Part model, mm, in its own coordinate system. Face numbers are marked on the shaded views. Coordinates: 2 decimals unless noted, no trailing zeros. Loops run counter-clockwise (first coordinate to the right, second up) from the corner with the lowest first, then second, coordinate; pieces in that order, holes last. Notation, with made-up numbers: (25, -38.75) - (52, -38.75) arc R37 ccw to (52, -0.75) - close; hole circle Ø3 at (79.5, 48). An arc over 180 degrees is marked (long way). Use a Markdown table: item, result. Add a question column.
1. Drop flat-ended pins along their axis: pin 1 (0.8 mm diameter, centred on x = -0.5, y = 17.5, fed in from -Z); pin 2 (4 mm diameter, centred on x = -45, z = 17.5, fed in from -Y); pin 3 (1 mm diameter, centred on x = 17, y = 8, fed in from +Z). Give the stop position or say it passes through.
2. Wall check: probe 1 along X at (y, z) = (4.25, 1.5); probe 2 along Y at (x, z) = (-23.5, -43.5); probe 3 along X at (y, z) = (2, -8). Give the ranges that are in metal, low to high. Write a range as [from, to].
3. Band-saw the part on A-A, the plane y = 10.5. Give the cut face in (x, z).
4. Pull direction Z, two halves, no side cores. Call the marked faces 1 and 2: pulls with the +Z half, pulls with the -Z half, needs draft (parallel to the pull), parting line crosses it, or undercut.
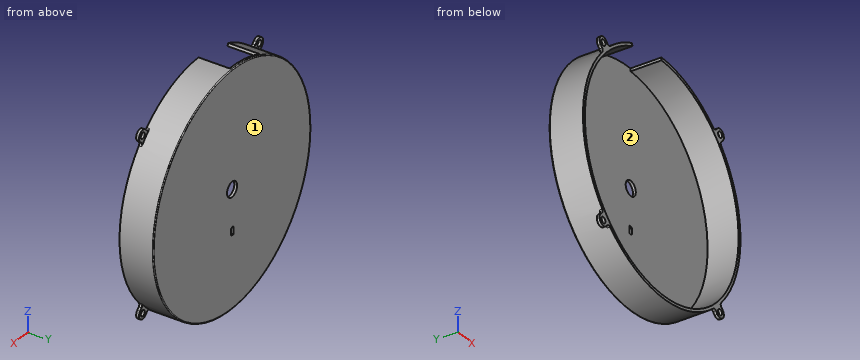
from build123d import *

# Parameters (mm, degrees)
EXTRUDE_1_DEPTH = 16.5
SKETCH_2_R      = 4
EXTRUDE_2_DEPTH = 1.5
FILLET_1_R      = 0.5
SKETCH_3_R      = 1.6
EXTRUDE_4_DEPTH = 1.5
FILLET_2_R      = 1.5


with BuildPart() as part:
    # Эскиз1 → Бобышка-Вытянуть1 (new body)
    with BuildSketch(Plane(origin=(0, 0, 0), x_dir=(1, 0, 0), z_dir=(0, 1, 0))):
        with BuildLine():
            Line((-23.77906371, -57.799706998), (-23.205036867, -56.41388361))
            ThreePointArc((-23.205036867, -56.41388361), (11.826941696, 59.842488669), (0, -61))
            Line((0, -61), (-0.15, -61))
            Line((-0.15, -61), (-0.15, -62.49982))
            ThreePointArc((-0.15, -62.49982), (12.193145126, 61.299080025), (-23.77906371, -57.799706998))
        make_face()
    extrude(amount=EXTRUDE_1_DEPTH)

    # Эскиз2 → Бобышка-Вытянуть2 (add)
    # profile 1 of 2: a face of its own
    with BuildSketch(Plane(origin=(0, 16.5, 0), x_dir=(1, 0, 0), z_dir=(0, 1, 0))):
        with BuildLine():
            Line((0, -61), (-0.15, -61))
            Line((-0.15, -61), (-0.15, -62.49982))
            ThreePointArc((-0.15, -62.49982), (12.193145126, 61.299080025), (-23.77906371, -57.799706998))
            Line((-23.77906371, -57.799706998), (-23.205036867, -56.41388361))
            ThreePointArc((-23.205036867, -56.41388361), (11.826941696, 59.842488669), (0, -61))
        make_face()
    # profile 2 of 2: a face of its own
    with BuildSketch(Plane(origin=(0, 16.5, 0), x_dir=(1, 0, 0), z_dir=(0, 1, 0))):
        with BuildLine():
            Line((-23.205036867, -56.41388361), (-23.77906371, -57.799706998))
            ThreePointArc((-23.77906371, -57.799706998), (-12.193145126, -61.299080025), (-0.15, -62.49982))
            Line((-0.15, -62.49982), (-0.15, -61))
            Line((-0.15, -61), (0, -61))
            ThreePointArc((0, -61), (11.826941696, 59.842488669), (-23.205036867, -56.41388361))
        make_face()
        with Locations(Location((0, 0, 0), (0, 0, 270))):
            Circle(SKETCH_2_R, mode=Mode.SUBTRACT)
        Polygon((-1, 23.5), (-1, 24.05), (-0.25, 24.05), (1, 23.5), (1, 20.3), (-0.25, 19.75), (-1, 19.75), (-1, 20.3), align=None, mode=Mode.SUBTRACT)
    extrude(amount=EXTRUDE_2_DEPTH)

    # Скругление1
    fillet_1_edges = [part.edges().sort_by_distance(p)[0] for p in [
        (23.77906371, 18, -57.799706998),
    ]]
    fillet(fillet_1_edges, radius=FILLET_1_R)

    # Эскиз3 → Бобышка-Вытянуть4 (add)
    # profile 1 of 4: a face of its own
    with BuildSketch(Plane.XZ):
        with BuildLine():
            Line((-42.021912433, 46.264553121), (-44.194173824, 48.436814511))
            ThreePointArc((-44.194173824, 48.436814511), (-48.436814511, 48.436814511), (-48.436814511, 44.194173824))
            Line((-48.436814511, 44.194173824), (-46.264553121, 42.021912433))
            ThreePointArc((-46.264553121, 42.021912433), (-44.194173824, 44.194173824), (-42.021912433, 46.264553121))
        make_face()
        with Locations(Location((-46.315494168, 46.315494168, 0), (0, 0, 270))):
            Circle(SKETCH_3_R, mode=Mode.SUBTRACT)
    # profile 2 of 4: a face of its own
    with BuildSketch(Plane.XZ):
        with BuildLine():
            Line((44.194173824, 48.436814511), (42.021912433, 46.264553121))
            ThreePointArc((42.021912433, 46.264553121), (44.194173824, 44.194173824), (46.264553121, 42.021912433))
            Line((46.264553121, 42.021912433), (48.436814511, 44.194173824))
            ThreePointArc((48.436814511, 44.194173824), (48.436814511, 48.436814511), (44.194173824, 48.436814511))
        make_face()
        with Locations(Location((46.315494168, 46.315494168, 0), (0, 0, 270))):
            Circle(SKETCH_3_R, mode=Mode.SUBTRACT)
    # profile 3 of 4: a face of its own
    with BuildSketch(Plane.XZ):
        with BuildLine():
            ThreePointArc((-42.021912433, -46.264553121), (-44.194173824, -44.194173824), (-46.264553121, -42.021912433))
            Line((-46.264553121, -42.021912433), (-48.436814511, -44.194173824))
            ThreePointArc((-48.436814511, -44.194173824), (-48.436814511, -48.436814511), (-44.194173824, -48.436814511))
            Line((-44.194173824, -48.436814511), (-42.021912433, -46.264553121))
        make_face()
        with Locations(Location((-46.315494168, -46.315494168, 0), (0, 0, 270))):
            Circle(SKETCH_3_R, mode=Mode.SUBTRACT)
    # profile 4 of 4: a face of its own
    with BuildSketch(Plane.XZ):
        with BuildLine():
            ThreePointArc((46.264553121, -42.021912433), (44.194173824, -44.194173824), (42.021912433, -46.264553121))
            Line((42.021912433, -46.264553121), (44.194173824, -48.436814511))
            ThreePointArc((44.194173824, -48.436814511), (48.436814511, -48.436814511), (48.436814511, -44.194173824))
            Line((48.436814511, -44.194173824), (46.264553121, -42.021912433))
        make_face()
        with Locations(Location((46.315494168, -46.315494168, 0), (0, 0, 270))):
            Circle(SKETCH_3_R, mode=Mode.SUBTRACT)
    extrude(amount=-EXTRUDE_4_DEPTH)

    # Скругление2
    fillet_2_edges = [part.edges().sort_by_distance(p)[0] for p in [
        (-42.021912433, 0.75, 46.264553121),
        (-46.264553121, 0.75, 42.021912433),
        (46.264553121, 0.75, 42.021912433),
        (42.021912433, 0.75, 46.264553121),
        (-46.264553121, 0.75, -42.021912433),
        (-42.021912433, 0.75, -46.264553121),
        (42.021912433, 0.75, -46.264553121),
        (46.264553121, 0.75, -42.021912433),
    ]]
    fillet(fillet_2_edges, radius=FILLET_2_R)


solid = part.part
Geometry check:
| question | item | result |
|---|---|---|
| 1 | pin 1 | stops at z = -62.5 |
| 1 | pin 2 | stops at y = 16.5 |
| 1 | pin 3 | stops at z = 60.28 |
| 2 | probe 1 | x = [-62.48, -60.98], [60.98, 62.48] |
| 2 | probe 2 | y = [16.5, 18] |
| 2 | probe 3 | x = [-61.99, -60.47], [60.47, 61.99] |
| 3 | outline | (-23.78, 57.8) arc R62.5 ccw (long way) to (-0.15, 62.5) - (-0.15, 61) - (0, 61) arc R61 cw (long way) to (-23.21, 56.41) - close |
| 4 | face 1 | needs draft |
| 4 | face 2 | undercut |
